```python
from build123d import *

# Parameters (mm, degrees)
SKETCH1_W                   = 107.1
SKETCH1_H                   = 6
SKETCH18_R                  = 6
BOSS_EXTRUDE1_DEPTH         = 72.5
CUT_EXTRUDE4_REACH          = 113.936
CUT_EXTRUDE4_END_RADIUS     = 6
CUT_EXTRUDE4_START          = -4.5
M5_TAPPED_HOLE3_D           = 4.2
M5_TAPPED_HOLE3_DEPTH       = 14
M5_TAPPED_HOLE3_CSINK_D     = 6
M5_TAPPED_HOLE3_CSINK_ANGLE = 90
M5_TAPPED_HOLE3_TIP         = 1.2618073
BOSS_EXTRUDE2_START         = 21.4
SKETCH22_R                  = 6
BOSS_EXTRUDE2_DEPTH         = 21.4
CHAMFER2_SIZE               = 1
SKETCH25_W                  = 3
SKETCH25_H                  = 3
CUT_EXTRUDE5_DEPTH          = 30
FILLET2_R                   = 1.5
SKETCH30_OUTSIDE_W          = 54.344
SKETCH30_OUTSIDE_H          = 54.344
SKETCH30_OUTSIDE_R          = 3
CUT_EXTRUDE10_DEPTH         = 12
CUT_EXTRUDE11_DEPTH         = 129.779850918
CUT_EXTRUDE11_DEPTH_BACK    = 129.779850918
SKETCH31_W                  = 5.87
SKETCH31_H                  = 22.819621357
SKETCH31_H_2                = 22.855520271
CUT_EXTRUDE12_START         = 4.5
CUT_EXTRUDE12_DEPTH         = 125.279850918
CUT_EXTRUDE13_START         = 50.3
SKETCH33_OUTSIDE_W          = 54.344
SKETCH33_OUTSIDE_H          = 54.344
SKETCH33_OUTSIDE_R          = 5.75
CUT_EXTRUDE13_DEPTH         = 1.5


with BuildPart() as part:
    # Sketch1 → Revolve1 (revolve)
    with BuildSketch(Plane(origin=(0, 0, 0), x_dir=(0, 0, -1), z_dir=(1, 0, 0)), mode=Mode.PRIVATE) as revolve1_sk:
        with Locations((53.55, 3)):
            Rectangle(SKETCH1_W, SKETCH1_H)
    revolve(revolve1_sk.sketch.rotate(Axis((0, 0, 38.636074766), (0, 0, -1)), 90), axis=Axis((0, 0, 38.636074766), (0, 0, -1)))

    # Sketch18 → Boss-Extrude1 (add)
    with BuildSketch(Plane.XY):
        Circle(SKETCH18_R)
    extrude(amount=BOSS_EXTRUDE1_DEPTH)

    # Cut-Extrude4: up to this cylinder (the profile starts inside it)
    cut_extrude4_end = Plane(origin=(0, 0, 57.9), z_dir=(0, 0, 1)) * Cylinder(CUT_EXTRUDE4_END_RADIUS, 240.872, mode=Mode.PRIVATE)
    # Sketch19 → Cut-Extrude4 (cut, up to the surface)
    with BuildSketch(Plane(origin=(0, 0, 0), x_dir=(1, 0, 0), z_dir=(0, 1, 0)).offset(CUT_EXTRUDE4_START), mode=Mode.PRIVATE) as cut_extrude4_sk1:
        with BuildLine():
            Line((-1.5, -63.9), (-1.5, -51.9))
            ThreePointArc((-1.5, -51.9), (0, -50.4), (1.5, -51.9))
            Line((1.5, -51.9), (1.5, -63.9))
            ThreePointArc((1.5, -63.9), (0, -65.4), (-1.5, -63.9))
        make_face()
    cut_extrude4_tool1 = extrude(cut_extrude4_sk1.sketch, amount=-CUT_EXTRUDE4_REACH, mode=Mode.PRIVATE) & cut_extrude4_end
    add(cut_extrude4_tool1.solids().sort_by_distance((0, -4.5, 57.9))[0], mode=Mode.SUBTRACT)

    # M5 Tapped Hole3
    with Locations(Plane.XY.offset(72.5)):
        with Locations((0, 0)):
            CounterSinkHole(M5_TAPPED_HOLE3_D / 2, M5_TAPPED_HOLE3_CSINK_D / 2, depth=M5_TAPPED_HOLE3_DEPTH, counter_sink_angle=M5_TAPPED_HOLE3_CSINK_ANGLE)
            with Locations((0, 0, -(M5_TAPPED_HOLE3_DEPTH + M5_TAPPED_HOLE3_TIP / 2))):  # 118° drill point
                Cone(0, M5_TAPPED_HOLE3_D / 2, M5_TAPPED_HOLE3_TIP, mode=Mode.SUBTRACT)

    # Sketch22 → Boss-Extrude2 (add)
    with BuildSketch(Plane(origin=(0, 0, -107.1), x_dir=(-1, 0, 0), z_dir=(0, 0, -1)).offset(BOSS_EXTRUDE2_START)):
        with Locations(Location((0, 0, 0), (0, 0, 180))):
            Circle(SKETCH22_R)
    extrude(amount=-BOSS_EXTRUDE2_DEPTH)

    # Chamfer2
    chamfer2_edges = [part.edges().sort_by_distance(p)[0] for p in [
        (-6, 0, 72.5),
    ]]
    chamfer(chamfer2_edges, length=CHAMFER2_SIZE)

    # Sketch25 → Cut-Extrude5 (cut)
    with BuildSketch(Plane.XY.offset(72.5)):
        with Locations((0, -6)):
            Rectangle(SKETCH25_W, SKETCH25_H)
    extrude(amount=-CUT_EXTRUDE5_DEPTH, mode=Mode.SUBTRACT)

    # Fillet2
    fillet2_edges = [part.edges().sort_by_distance(p)[0] for p in [
        (1.5, -5.15473751, 42.5),
        (-1.5, -5.15473751, 42.5),
    ]]
    fillet(fillet2_edges, radius=FILLET2_R - 0.0001)  # a hair under: the kernel refuses the full size

    # Sketch30 outside → Cut-Extrude10 (cut)
    with BuildSketch(Plane(origin=(0, 0, -128.5), x_dir=(-1, 0, 0), z_dir=(0, 0, -1))):
        Rectangle(SKETCH30_OUTSIDE_W, SKETCH30_OUTSIDE_H)
        Circle(SKETCH30_OUTSIDE_R, mode=Mode.SUBTRACT)
    extrude(amount=-CUT_EXTRUDE10_DEPTH, mode=Mode.SUBTRACT)

    # Sketch31 → Cut-Extrude11 (cut, two sides: drawn at the far end of the back side and taken through both)
    with BuildSketch(Plane(origin=(0, 0, 0), x_dir=(0, 0, -1), z_dir=(1, 0, 0)).offset(-CUT_EXTRUDE11_DEPTH_BACK)):
        with Locations((101.365, -16.709810679)):
            Rectangle(SKETCH31_W, SKETCH31_H)
        with Locations((101.365, 16.727760135)):
            Rectangle(SKETCH31_W, SKETCH31_H_2)
    extrude(amount=CUT_EXTRUDE11_DEPTH + CUT_EXTRUDE11_DEPTH_BACK, mode=Mode.SUBTRACT)

    # Sketch32 → Cut-Extrude12 (cut, through all)
    with BuildSketch(Plane(origin=(0, 0, 0), x_dir=(0, 0, -1), z_dir=(1, 0, 0)).offset(CUT_EXTRUDE12_START)):
        with BuildLine():
            Line((107.365, -1.5), (95.365, -1.5))
            ThreePointArc((95.365, -1.5), (93.865, 0), (95.365, 1.5))
            Line((95.365, 1.5), (107.365, 1.5))
            ThreePointArc((107.365, 1.5), (108.865, 0), (107.365, -1.5))
        make_face()
    extrude(amount=CUT_EXTRUDE12_DEPTH, mode=Mode.SUBTRACT)

    # Sketch33 outside → Cut-Extrude13 (cut)
    with BuildSketch(Plane(origin=(0, 0, 41.3), x_dir=(-1, 0, 0), z_dir=(0, 0, -1)).offset(CUT_EXTRUDE13_START)):
        Rectangle(SKETCH33_OUTSIDE_W, SKETCH33_OUTSIDE_H)
        Circle(SKETCH33_OUTSIDE_R, mode=Mode.SUBTRACT)
    extrude(amount=-CUT_EXTRUDE13_DEPTH, mode=Mode.SUBTRACT)


solid = part.part
```
Input: part model. Units: mm. Frame: model coordinates. A direction names the side the tool comes from. Coordinates: 2 decimals unless noted, no trailing zeros. Write each loop counter-clockwise with the first axis right and the second up, starting at its lowest first coordinate (ties: lowest second). Pieces come first, ordered by that corner, then holes.
1) Set-up query: faces 1 (the cylindrical face through (-2.003, 0.631, 64.958)), 2 (the flat face through (3, -1, -116.5)), 3 (the flat face through (0, -5.3, -101)). Return all of +Z, -Z, +X, -X, +Y, -Y with unobstructed straight access to the full face (end or side cutting, diameter ignored); none if empty.
2) Section A-A on z = 21. Output: boundary loops of the cut face in (x, y).
3) Mould query, pull axis X, two halves, no side actions, for faces 4 (the conical face through (0.34, -0.14, 57.46)), 5 (the flat face through (0, 5.3, -101)), 6 (the cylindrical face through (0.75, 5.7, -8.26)). Classes: pulls with the +X half, pulls with the -X half, needs draft (parallel to the pull), parting line crosses it, or undercut.
4) Material intervals for line 1 along X through (y, z) = (0, 67); line 2 along Y through (x, z) = (0, 66); line 3 along Y through (x, z) = (-0.5, 56), sorted ascending.
5) Pin query (flat end, axial travel): pin 1 Ø0.6 at (x, y) = (0, 5.5) entering from +Z; pin 2 Ø1 at (x, z) = (5, -100) entering from +Y; pin 3 Ø0.6 at (x, y) = (0.5, 5.5) entering from -Z. Return the tip coordinate at first contact, or that it passes through.
Check result:
1. face 1: +Z
1. face 2: -Z
1. face 3: +X, -X, -Y
2. outline: circle Ø12 at (0, 0)
3. face 4: undercut
3. face 5: needs draft
3. face 6: parting line crosses it
4. line 1: x = -6 to -2.1, 2.1 to 6
4. line 2: y = -4.5 to -2.1, 2.1 to 6
4. line 3: y = -4.5 to 5.98
5. pin 1: stops at z = 72.3
5. pin 2: stops at y = 3.97
5. pin 3: stops at z = -116.5
